Source: CAD feature listing. Evaluate the final solid. Frame: model axes, mm. A direction names the side the tool comes from. Round coordinates to 2 decimals unless told otherwise and drop trailing zeros. Loops run counter-clockwise (first coordinate to the right, second up) from the corner with the lowest first, then second, coordinate; pieces in that order, holes last. Notation, with made-up numbers: (15.25, 69.5) -> (66.25, 69.5) arc R33 cw to (66.25, 101.5) -> close; hole circle Ø5 at (74, -32). An arc over 180 degrees is marked (long way). Write item = value, one per line.
from build123d import *

# Parameters (mm, degrees)
IZIM1_R                     = 6
Y_KSEKLIK_EKSTR_ZYON1_DEPTH = 10
Y_KSEKLIK_EKSTR_ZYON2_DEPTH = 5
FEDER1_REACH                = 103.716
IZIM5_WALL_W                = 245.79202862
IZIM5_WALL_H                = 5
FEDER8_REACH                = 103.716
IZIM6_WALL_W                = 245.79202862
IZIM6_WALL_H                = 5


with BuildPart() as part:
    # Çizim1 → Yükseklik-Ekstrüzyon1 (new body)
    with BuildSketch(Plane(origin=(0, 0, 0), x_dir=(1, 0, 0), z_dir=(0, 1, 0))):
        with BuildLine():
            Line((-142.676154711, -27.016601459), (-52.676154711, -27.016601459))
            ThreePointArc((-52.676154711, -27.016601459), (-49.140620805, -28.481067553), (-47.676154711, -32.016601459))
            Line((-47.676154711, -32.016601459), (-47.676154711, -57.016601459))
            ThreePointArc((-47.676154711, -57.016601459), (-49.140620805, -60.552135365), (-52.676154711, -62.016601459))
            Line((-52.676154711, -62.016601459), (-142.676154711, -62.016601459))
            ThreePointArc((-142.676154711, -62.016601459), (-146.211688617, -60.552135365), (-147.676154711, -57.016601459))
            Line((-147.676154711, -57.016601459), (-147.676154711, -32.016601459))
            ThreePointArc((-147.676154711, -32.016601459), (-146.211688617, -28.481067553), (-142.676154711, -27.016601459))
        make_face()
        with Locations(Location((-133.676154711, -44.516601459, 0), (0, 0, 270))):
            Circle(IZIM1_R, mode=Mode.SUBTRACT)
        with Locations(Location((-61.676154711, -44.516601459, 0), (0, 0, 270))):
            Circle(IZIM1_R, mode=Mode.SUBTRACT)
    extrude(amount=Y_KSEKLIK_EKSTR_ZYON1_DEPTH)

    # Çizim3 → Yükseklik-Ekstrüzyon2 (add)
    with BuildSketch(Plane.XY.offset(62.016601459)):
        with BuildLine():
            Line((-117.676154711, 40), (-117.676154711, 10))
            Line((-117.676154711, 10), (-77.676154711, 10))
            Line((-77.676154711, 10), (-77.676154711, 40))
            Line((-77.676154711, 40), (-92.676154711, 40))
            Line((-92.676154711, 40), (-92.676154711, 29))
            ThreePointArc((-92.676154711, 29), (-97.676154711, 23.936325368), (-102.676154711, 29))
            Line((-102.676154711, 29), (-102.676154711, 40))
            Line((-102.676154711, 40), (-117.676154711, 40))
        make_face()
    extrude(amount=-Y_KSEKLIK_EKSTR_ZYON2_DEPTH)

    # Çizim5 wall → Feder1 (add, up to next)
    with BuildSketch(Plane(origin=(-77.676154711, 25, 43.516601459), x_dir=(0, -0.743294146247, -0.668964731622), z_dir=(0, 0.668964731622, -0.743294146247)), mode=Mode.PRIVATE) as feder1_sk1:
        with Locations((0, 2.5)):
            Rectangle(IZIM5_WALL_W, IZIM5_WALL_H)
    feder1_tool1 = extrude(feder1_sk1.sketch, amount=-FEDER1_REACH, mode=Mode.PRIVATE) - part.part
    add(feder1_tool1.solids().sort_by_distance((-77.676154711, 25, 43.516601459))[0])

    # Çizim6 wall → Feder8 (add, up to next)
    with BuildSketch(Plane(origin=(-117.676154711, 25, 43.516601459), x_dir=(0, -0.743294146247, -0.668964731622), z_dir=(0, -0.668964731622, 0.743294146247)), mode=Mode.PRIVATE) as feder8_sk1:
        with Locations((0, 2.5)):
            Rectangle(IZIM6_WALL_W, IZIM6_WALL_H)
    feder8_tool1 = extrude(feder8_sk1.sketch, amount=FEDER8_REACH, mode=Mode.PRIVATE) - part.part
    add(feder8_tool1.solids().sort_by_distance((-117.676154711, 25, 43.516601459))[0])


solid = part.part
1. Section query D-D (x = -84.5). Return the cut outline in (y, z), then the cut area to 3 significant figures.
Evaluation:
outline = (0, 27.02) -> (10, 27.02) -> (10, 57.02) -> (40, 57.02) -> (40, 62.02) -> (0, 62.02) -> close
area = 500 mm²
2. Section query C-C (y = 34.5). Return the cut outline in (x, z), then the cut area to 4 significant figures.
Evaluation:
outline = (-117.68, 52.07) -> (-112.68, 52.07) -> (-112.68, 57.02) -> (-102.68, 57.02) -> (-102.68, 62.02) -> (-117.68, 62.02) -> close; (-92.68, 57.02) -> (-82.68, 57.02) -> (-82.68, 52.07) -> (-77.68, 52.07) -> (-77.68, 62.02) -> (-92.68, 62.02) -> close
area = 199.5 mm²
3. Contact query for flat-ended pins moving along their axis: pin 1 Ø1 at (x, z) = (-101.5, 50.5) entering from +Y; pin 2 Ø9 at (y, z) = (30, 47.5) entering from -X; pin 3 Ø1 at (x, y) = (-100.5, 13) entering from -Z; pin 4 Ø12 at (x, y) = (-124.5, 31) entering from -Z. Output: stop coordinate, or through.
Evaluation:
pin_1 = 10
pin_2 = -117.68
pin_3 = 57.02
pin_4 = through
4. Set-up query: faces 4 (the face through (-117.676, 20, 52)), 5 (the face through (-102.676, 34, 60)), 6 (the face through (-82.676, 22, 48)). Return all of +Z, -Z, +X, -X, +Y, -Y with unobstructed straight access to the full face (end or side cutting, diameter ignored); none if empty.
Evaluation:
face_4 = +Z, -Z, -X, +Y
face_5 = +Z, -Z, +Y
face_6 = -Z, +Y
5. Section query A-A (x = -64.5). Return the cut outline in (y, z).
Evaluation:
outline = (0, 27.02) -> (10, 27.02) -> (10, 39.22) -> (0, 39.22) -> close; (0, 49.81) -> (10, 49.81) -> (10, 62.02) -> (0, 62.02) -> close
6. Section query B-B (z = 41). Return the cut outline in (x, y), then the cut area to 3 significant figures.
Evaluation:
outline = (-147.68, 0) -> (-138.54, 0) -> (-138.54, 10) -> (-147.68, 10) -> close; (-128.81, 0) -> (-66.54, 0) -> (-66.54, 10) -> (-77.68, 10) -> (-77.68, 22.2) -> (-82.68, 22.2) -> (-82.68, 10) -> (-112.68, 10) -> (-112.68, 22.2) -> (-117.68, 22.2) -> (-117.68, 10) -> (-128.81, 10) -> close; (-56.81, 0) -> (-47.68, 0) -> (-47.68, 10) -> (-56.81, 10) -> close
area = 928 mm²
7. Line query: probe 1 along X at (y, z) = (33.5, 61); probe 2 along X at (y, z) = (7, 43.5); probe 3 along X at (y, z) = (15.5, 39.5). Output: solid intervals per line, ascending. Write a range as from..to.
Evaluation:
probe_1 = -117.68..-102.68, -92.68..-77.68
probe_2 = -147.68..-139.59, -127.76..-67.59, -55.76..-47.68
probe_3 = -117.68..-112.68, -82.68..-77.68
8. Mould query, pull axis X, two halves, no side actions, for faces 1 (the face through (-92.676, 35, 60)), 2 (the face through (-77.676, 20, 52)), 3 (the face through (-97, 0, 44)). Classes: released by +X, released by -X, zero draft, split by the parting line, or undercut.
Evaluation:
face_1 = undercut
face_2 = released by +X
face_3 = zero draft
